The listing builds one solid part. Answer for the finished solid, in the listing's coordinates (mm). A direction names the side the tool comes from. Coordinates: 2 decimals unless noted, no trailing zeros. Order: outer loops, then holes, each group sorted by start corner. A loop starts at its lowest first (then second) coordinate and runs counter-clockwise, first axis right, second up. Notation, with made-up numbers: (46.25, -8) -> (79.25, -8) arc R14 cw to (79.25, 12) -> close; hole circle Ø5 at (38.5, 82). An arc over 180 degrees is marked (long way). One line per question, with ' | ' between items.
from build123d import *

# Parameters (mm, degrees)
SKETCH1_R           = 57.5
SKETCH1_R_2         = 55.5
BOSS_EXTRUDE1_DEPTH = 5


with BuildPart() as part:
    # Sketch1 → Boss-Extrude1 (new body)
    # profile 1 of 3: a face of its own
    with BuildSketch(Plane.XY):
        with BuildLine():
            ThreePointArc((-56.86052693, -8.551635942), (-57.33990887, -4.287755914), (-57.5, 0))
            Line((-57.5, 0), (-57.5, 57.5))
            Line((-57.5, 57.5), (-98.518106022, 57.5))
            Line((-98.518106022, 57.5), (-98.518106022, 50.5))
            Line((-98.518106022, 50.5), (-62.662833113, 50.5))
            Line((-62.662833113, 50.5), (-62.662833113, 0.474482067))
            Line((-62.662833113, 0.474482067), (-56.86052693, -8.551635942))
        make_face()
    # profile 2 of 3: a face of its own
    with BuildSketch(Plane.XY):
        Circle(SKETCH1_R)
        Circle(SKETCH1_R_2, mode=Mode.SUBTRACT)
    # profile 3 of 3: a face of its own
    with BuildSketch(Plane.XY):
        with BuildLine():
            Line((57.5, 57.5), (57.5, 0))
            ThreePointArc((57.5, 0), (57.33990887, -4.287755914), (56.86052693, -8.551635942))
            Line((56.86052693, -8.551635942), (62.662833113, 0.474482067))
            Line((62.662833113, 0.474482067), (62.662833113, 50.5))
            Line((62.662833113, 50.5), (98.518106022, 50.5))
            Line((98.518106022, 50.5), (98.518106022, 57.5))
            Line((98.518106022, 57.5), (57.5, 57.5))
        make_face()
    extrude(amount=BOSS_EXTRUDE1_DEPTH)


solid = part.part
Item 1: Section A-A, the plane x = 0 is taken. Give the vertices of the cut face in (y, z).
Computed values:
outline: (-57.5, 0) -> (-55.5, 0) -> (-55.5, 5) -> (-57.5, 5) -> close; (55.5, 0) -> (57.5, 0) -> (57.5, 5) -> (55.5, 5) -> close
Item 2: Section C-C, the plane z = 1.9 is taken. Give the vertices of the cut face in (x, y).
Computed values:
outline: (-98.52, 50.5) -> (-62.66, 50.5) -> (-62.66, 0.47) -> (-56.86, -8.55) arc R57.5 ccw to (56.86, -8.55) -> (62.66, 0.47) -> (62.66, 50.5) -> (98.52, 50.5) -> (98.52, 57.5) -> (57.5, 57.5) -> (57.5, 0) arc R57.5 ccw to (-57.5, 0) -> (-57.5, 57.5) -> (-98.52, 57.5) -> close; hole circle Ø111 at (0, 0)
Item 3: Section D-D, the plane y = -11 is taken. Give the vertices of the cut face in (x, z).
Computed values:
outline: (-56.44, 0) -> (-54.4, 0) -> (-54.4, 5) -> (-56.44, 5) -> close; (54.4, 0) -> (56.44, 0) -> (56.44, 5) -> (54.4, 5) -> close
Item 4: Determine the mould class of faces 1 (the face through (1.264, 57.486, 2.465)), 2 (the face through (0, 56, 5)), 3 (the face through (59.72, -4.1, 2.46)), 4 (the face through (52.937, 16.671, 2.465)) for opening direction X: pulls with the +X half, pulls with the -X half, needs draft (parallel to the pull), parting line crosses it, or undercut.
Computed values:
face 1: undercut | face 2: needs draft | face 3: pulls with the +X half | face 4: undercut
Item 5: Each of these flat-tipped pins is pushed along its axis until it touches: pin 1 Ø1.5 at (y, z) = (-22.5, 1) entering from -X; pin 2 Ø2.5 at (x, z) = (-78, 3) entering from -Y; pin 3 Ø1.5 at (y, z) = (41.5, 3) entering from +X. Where does it stop, or does it pass through?
Computed values:
pin 1: stops at x = -53.23 | pin 2: stops at y = 50.5 | pin 3: stops at x = 62.66
Item 6: Section B-B, the plane y = 15 is taken. Give the vertices of the cut face in (x, z).
Computed values:
outline: (-62.66, 0) -> (-57.5, 0) -> (-57.5, 5) -> (-62.66, 5) -> close; (-55.51, 0) -> (-53.43, 0) -> (-53.43, 5) -> (-55.51, 5) -> close; (53.43, 0) -> (55.51, 0) -> (55.51, 5) -> (53.43, 5) -> close; (57.5, 0) -> (62.66, 0) -> (62.66, 5) -> (57.5, 5) -> close
Item 7: For faces 5 (the face through (-1.14, -57.49, 2.46)), 6 (the face through (-62.663, 26, 2)), 7 (the face through (62.663, 25, 2)), determine the directions among +Z, -Z, +X, -X, +Y, -Y from which every point of the face is accessible in a straight line to the end or side of a thin tool.
Computed values:
face 5: +Z, -Z, -Y | face 6: +Z, -Z, -X, -Y | face 7: +Z, -Z, +X, -Y
Item 8: Find the intervals of material crossed by L1, parallel to Y at x = 0, z = 2.7; L2, parallel to X at y = 36, z = 4.8; L3, parallel to X at y = 37, z = 0.3, in increasing order.
Computed values:
L1: y = -57.5 to -55.5, 55.5 to 57.5 | L2: x = -62.66 to -57.5, -44.84 to -42.24, 42.24 to 44.84, 57.5 to 62.66 | L3: x = -62.66 to -57.5, -44.01 to -41.37, 41.37 to 44.01, 57.5 to 62.66
